from build123d import *

# Parameters (mm, degrees)
REDONDEO1_R          = 0.2
CHAFL_N1_SIZE        = 0.3
CHAFL_N2_SIZE        = 0.5
CORTAR_BARRER1_START = 3.956316317
CORTAR_BARRER1_DEPTH = 1.043683683


with BuildPart() as part:
    # Croquis1 → Revolución1 (revolve)
    with BuildSketch(Plane.XY):
        Polygon((0, 0), (0, -45), (2.5, -45), (2.5, 0), (4.25, 0), (4.25, 5), (0, 5), align=None)
    revolve(axis=Axis((0, -1001.198752701, 0), (0, 1, 0)))

    # Redondeo1
    redondeo1_edges = [part.edges().sort_by_distance(p)[0] for p in [
        (-2.5, 0, 0),
    ]]
    fillet(redondeo1_edges, radius=REDONDEO1_R)

    # Chaflán1
    chafl_n1_edges = [part.edges().sort_by_distance(p)[0] for p in [
        (-2.5, -45, 0),
    ]]
    chamfer(chafl_n1_edges, length=CHAFL_N1_SIZE)

    # Chaflán2
    chafl_n2_edges = [part.edges().sort_by_distance(p)[0] for p in [
        (-4.25, 5, 0),
        (-4.25, 0, 0),
    ]]
    chamfer(chafl_n2_edges, length=CHAFL_N2_SIZE)

    # Cortar-Barrer1: read off the stored shape, not the designer's step
    # Cortar-Barrer1 outline → Cortar-Barrer1 (cut)
    with BuildSketch(Plane(origin=(0, 0, 0), x_dir=(1, 0, 0), z_dir=(0, 1, 0)).offset(CORTAR_BARRER1_START)):
        Polygon((1.154700538, 2), (-1.154700538, 2), (-2.309401077, 0), (-1.154700538, -2), (1.154700538, -2), (2.309401077, 0), align=None)
    extrude(amount=CORTAR_BARRER1_DEPTH, mode=Mode.SUBTRACT)

    # Cortar-Barrer1 2: loft between two sections, ruled curve by curve
    cortar_barrer1_2_from = [
        Edge.make_line((-2.309401077, 3.956316317, 0), (-1.154700538, 3.956316317, -2)),
        Edge.make_line((-1.154700538, 3.956316317, 2), (-2.309401077, 3.956316317, 0)),
        Edge.make_line((-1.154700538, 3.956316317, -2), (1.154700538, 3.956316317, -2)),
        Edge.make_line((1.154700538, 3.956316317, 2), (-1.154700538, 3.956316317, 2)),
        Edge.make_line((1.154700538, 3.956316317, -2), (2.309401077, 3.956316317, 0)),
        Edge.make_line((2.309401077, 3.956316317, 0), (1.154700538, 3.956316317, 2)),
    ]
    cortar_barrer1_2_to = [
        Edge.make_line((-1.235376897, 3.257522104, 0), (-0.617688448, 3.257522104, -1.069867776)),
        Edge.make_line((-0.617688448, 3.257522104, 1.069867776), (-1.235376897, 3.257522104, 0)),
        Edge.make_line((-0.617688448, 3.257522104, -1.069867776), (0.617688448, 3.257522104, -1.069867776)),
        Edge.make_line((0.617688448, 3.257522104, 1.069867776), (-0.617688448, 3.257522104, 1.069867776)),
        Edge.make_line((0.617688448, 3.257522104, -1.069867776), (1.235376897, 3.257522104, 0)),
        Edge.make_line((1.235376897, 3.257522104, 0), (0.617688448, 3.257522104, 1.069867776)),
    ]
    cortar_barrer1_2 = Solid(Shell([*[Face.make_surface_from_curves(cortar_barrer1_2_from[k], cortar_barrer1_2_to[k]) for k in range(6)], Face(Wire(cortar_barrer1_2_from)), Face(Wire(cortar_barrer1_2_to))]))
    add(cortar_barrer1_2, mode=Mode.SUBTRACT)


solid = part.part
Geometry check sheet. Reference: the model listing, model coordinates, mm. A direction names the side the tool comes from. Give positions to 0.01 mm unless a question says otherwise; leave off trailing zeros. Write each loop counter-clockwise with the first axis right and the second up, starting at its lowest first coordinate (ties: lowest second). Pieces come first, ordered by that corner, then holes. Notation, with made-up numbers: (-3.5, -32) - (23.5, -32) arc R14 cw to (23.5, -24) - close; hole circle Ø10 at (-27, -1). An arc over 180 degrees is marked (long way). Put each result on its own line as item: value.
1. Sectioned sample at A-A, the plane y = -34.5. Enter the section's corners in (x, z), plus the area to 3 significant figures.
Ans:
outline: circle Ø5 at (0, 0)
area: 19.6 mm²
2. Sectioned sample at B-B, the plane y = 1. Enter the section's corners in (x, z), plus the area to 3 significant figures.
Ans:
outline: circle Ø8.5 at (0, 0)
area: 56.7 mm²
3. Set-up check for faces 4 (the flat face through (2, 5, 2)), 5 (the cylindrical face through (-0.54, -22.14, 2.44)), 6 (the flat face through (-1.724, 4.471, -1.014)): record each of +Z, -Z, +X, -X, +Y, -Y from which the full face is reachable in a straight line by a thin tool's end or side.
Ans:
face 4: +Z, -Z, +X, -X, +Y
face 5: -Y
face 6: +Y
4. Draft check along X on faces 1 (the flat face through (1.74, 4.47, -0.99)), 2 (the cylindrical face through (2.285, 2.528, -3.584)), 3 (the flat face through (1, 0, -3)). Enter one of: +X half, -X half, draft (parallel to the pull), parting line (faces both ways), or undercut.
Ans:
face 1: undercut
face 2: parting line
face 3: draft
5. Thickness scan on line 1 (Y direction, x = -0.5, z = 3.5); line 2 (Z direction, x = -1.5, y = -28.5); line 3 (Y direction, x = 0, z = -0.75). Record the ranges inside material, lowest first.
Ans:
line 1: y = 0 to 5
line 2: z = -2 to 2
line 3: y = -45 to 3.26
6. Go/stop test with flat-tipped pins: pin 1 (5 mm diameter, centred on y = -17.5, z = 2.5, fed in from +X); pin 2 (5 mm diameter, centred on x = -1, y = -16, fed in from +Z); pin 3 (1.7 mm diameter, centred on x = 0, z = 0, fed in from +Y). Record where each tip stops, or that it passes through.
Ans:
pin 1: stops at x = 2.5
pin 2: stops at z = 2.5
pin 3: stops at y = 3.26
